from build123d import *

# Parameters (mm, degrees)
ESQUISSE1_W                  = 70
ESQUISSE1_H                  = 70
EXTRUSION1_DEPTH             = 5
CHANFREIN1_SIZE              = 5
EXTRUSION2_DEPTH             = 23
EXTRUSION2_DEPTH_BACK        = 5
ESQUISSE2_W                  = 5
ESQUISSE2_H                  = 40
ESQUISSE3_R                  = 3
ENL_V_MAT_EXTRU_1_DEPTH      = 82.572054038
ESQUISSE4_R                  = 12
ENL_V_MAT_EXTRU_2_DEPTH      = 61.074953184
ESQUISSE5_R                  = 23.5
ENL_V_MAT_EXTRU_3_DEPTH      = 2
ESQUISSE6_R                  = 2.25
ENL_V_MAT_EXTRU_4_DEPTH      = 61.074953184
R_P_TITION_CIRCULAIRE1_COUNT = 4


with BuildPart() as part:
    # Esquisse1 → Extrusion1 (new body)
    with BuildSketch(Plane.XY):
        Rectangle(ESQUISSE1_W, ESQUISSE1_H)
        with BuildLine():
            Line((-22, 32.75), (25, 32.75))
            ThreePointArc((25, 32.75), (27.75, 30), (25, 27.25))
            Line((25, 27.25), (-22, 27.25))
            ThreePointArc((-22, 27.25), (-24.75, 30), (-22, 32.75))
        make_face(mode=Mode.SUBTRACT)
        with BuildLine():
            Line((-22, -27.25), (25, -27.25))
            ThreePointArc((25, -27.25), (27.75, -30), (25, -32.75))
            Line((25, -32.75), (-22, -32.75))
            ThreePointArc((-22, -32.75), (-24.75, -30), (-22, -27.25))
        make_face(mode=Mode.SUBTRACT)
    extrude(amount=EXTRUSION1_DEPTH)

    # Chanfrein1
    chanfrein1_edges = [part.edges().sort_by_distance(p)[0] for p in [
        (-35, 35, 2.5),
        (35, 35, 2.5),
        (35, -35, 2.5),
        (-35, -35, 2.5),
    ]]
    chamfer(chanfrein1_edges, length=CHANFREIN1_SIZE)

    # Esquisse2 → Extrusion2 (add, two sides: drawn at the far end of the back side and taken through both)
    with BuildSketch(Plane(origin=(0, 0, 0), x_dir=(-1, 0, 0), z_dir=(0, 0, -1)).offset(-EXTRUSION2_DEPTH_BACK)):
        with Locations((37.5, 0)):
            Rectangle(ESQUISSE2_W, ESQUISSE2_H)
    extrude(amount=EXTRUSION2_DEPTH + EXTRUSION2_DEPTH_BACK)

    # Esquisse3 → Enlèv. mat.-Extru.1 (cut, through all)
    with BuildSketch(Plane(origin=(-35, 0, 0), x_dir=(0, 0, -1), z_dir=(1, 0, 0))):
        with Locations((14, 0)):
            Circle(ESQUISSE3_R)
    extrude(amount=-ENL_V_MAT_EXTRU_1_DEPTH, mode=Mode.SUBTRACT)

    # Esquisse4 → Enlèv. mat.-Extru.2 (cut, through all)
    with BuildSketch(Plane.XY.offset(5)):
        Circle(ESQUISSE4_R)
    extrude(amount=-ENL_V_MAT_EXTRU_2_DEPTH, mode=Mode.SUBTRACT)

    # Esquisse5 → Enlèv. mat.-Extru.3 (cut)
    with BuildSketch(Plane(origin=(0, 0, 0), x_dir=(-1, 0, 0), z_dir=(0, 0, -1))):
        Circle(ESQUISSE5_R)
    extrude(amount=-ENL_V_MAT_EXTRU_3_DEPTH, mode=Mode.SUBTRACT)

    # Esquisse6 → Enlèv. mat.-Extru.4 (cut, through all)
    with BuildSketch(Plane.XY.offset(5)):
        with Locations((0, -17.5)):
            Circle(ESQUISSE6_R)
    enl_v_mat_extru_4 = extrude(amount=-ENL_V_MAT_EXTRU_4_DEPTH, mode=Mode.SUBTRACT)

    # Répétition circulaire1: Enlèv. mat.-Extru.4 ×4 about axis
    r_p_tition_circulaire1_axis = Axis((0, 0, 0), (0, 0, 1))
    for i in range(1, R_P_TITION_CIRCULAIRE1_COUNT):
        add(enl_v_mat_extru_4.rotate(r_p_tition_circulaire1_axis, i * 360 / R_P_TITION_CIRCULAIRE1_COUNT), mode=Mode.SUBTRACT)


solid = part.part
Read the model definition and answer for the solid it produces. Units are mm, in the model's axes. A direction names the side the tool comes from. Round coordinates to 2 decimals unless told otherwise and drop trailing zeros. Loops run counter-clockwise (first coordinate to the right, second up) from the corner with the lowest first, then second, coordinate; pieces in that order, holes last. Notation, with made-up numbers: (15, -36.75) - (30, -36.75) arc R25 cw to (30, 0.25) - close; hole circle Ø3 at (36.5, 67.25). An arc over 180 degrees is marked (long way). One line per question, with ' | ' between items. Start each with the question number.
Q1. For faces 1 (the flat face through (-24, 0, 0)), 2 (the cylindrical face through (-24.75, -30.06, 2.46)), 3 (the flat face through (-35, 25, 2)), determine the directions among +Z, -Z, +X, -X, +Y, -Y from which every point of the face is accessible in a straight line to the end or side of a thin tool.
Q2. Flat-ended cylindrical pins translate along their axes: pin 1 (5 mm diameter, centred on y = 0, z = -14, fed in from +X); pin 2 (2 mm diameter, centred on x = -29.5, y = 23.5, fed in from -Z); pin 3 (5.5 mm diameter, centred on y = -25, z = 3, fed in from -X); pin 4 (2.5 mm diameter, centred on x = -36.5, z = -5.5, fed in from -Y). Find the tip coordinate at first contact, or state that the pin passes through.
Q3. Find the intervals of material crossed by L1, parallel to Y at x = 17.5, z = 3.1; L2, parallel to Y at x = -21.5, z = 3; L3, parallel to Y at x = 0, z = 4.4, in increasing order.
Q4. Section D-D on x = 13 is taken. Give the vertices of the cut face in (y, z), plus the area to 3 significant figures.
Q5. Section B-B on z = -14 is taken. Give the vertices of the cut face in (x, y).
Q6. Section C-C on y = 0 is taken. Give the vertices of the cut face in (x, z).
Q7. Section A-A on x = 0 is taken. Give the vertices of the cut face in (y, z).
Q8. For a pull along Y with two mould halves and no side action, classify faces 4 (the cylindrical face through (-24.75, 29.94, 2.46)), 5 (the flat face through (-37, -20, -9)), 6 (the flat face through (35, 0, 2)), 7 (the flat face through (33, 32, 2)) as +Y half, -Y half, draft (parallel to the pull), parting line (faces both ways), or undercut.
Established:
1) face 1: -Z, +X, +Y, -Y | face 2: +Z, -Z | face 3: +Z, -Z, -X, +Y
2) pin 1: through | pin 2: z = 0 | pin 3: x = -35 | pin 4: y = -20
3) L1: -35 to -32.75, -27.25 to -2.25, 2.25 to 27.25, 32.75 to 35 | L2: -35 to -32.75, -27.25 to 27.25, 32.75 to 35 | L3: -35 to -32.75, -27.25 to -19.75, -15.25 to -12, 12 to 15.25, 19.75 to 27.25, 32.75 to 35
4) outline: (-35, 0) - (-32.75, 0) - (-32.75, 5) - (-35, 5) - close; (-27.25, 0) - (-19.58, 0) - (-19.58, 2) - (19.58, 2) - (19.58, 0) - (27.25, 0) - (27.25, 5) - (-27.25, 5) - close; (32.75, 0) - (35, 0) - (35, 5) - (32.75, 5) - close | area: 217 mm²
5) outline: (-40, -20) - (-35, -20) - (-35, -3) - (-40, -3) - close; (-40, 3) - (-35, 3) - (-35, 20) - (-40, 20) - close
6) outline: (-40, -23) - (-35, -23) - (-35, -17) - (-40, -17) - close; (-40, -11) - (-35, -11) - (-35, 0) - (-23.5, 0) - (-23.5, 2) - (-19.75, 2) - (-19.75, 5) - (-40, 5) - close; (-15.25, 2) - (-12, 2) - (-12, 5) - (-15.25, 5) - close; (12, 2) - (15.25, 2) - (15.25, 5) - (12, 5) - close; (19.75, 2) - (23.5, 2) - (23.5, 0) - (35, 0) - (35, 5) - (19.75, 5) - close
7) outline: (-35, 0) - (-32.75, 0) - (-32.75, 5) - (-35, 5) - close; (-27.25, 0) - (-23.5, 0) - (-23.5, 2) - (-19.75, 2) - (-19.75, 5) - (-27.25, 5) - close; (-15.25, 2) - (-12, 2) - (-12, 5) - (-15.25, 5) - close; (12, 2) - (15.25, 2) - (15.25, 5) - (12, 5) - close; (19.75, 2) - (23.5, 2) - (23.5, 0) - (27.25, 0) - (27.25, 5) - (19.75, 5) - close; (32.75, 0) - (35, 0) - (35, 5) - (32.75, 5) - close
8) face 4: undercut | face 5: -Y half | face 6: draft | face 7: +Y half
